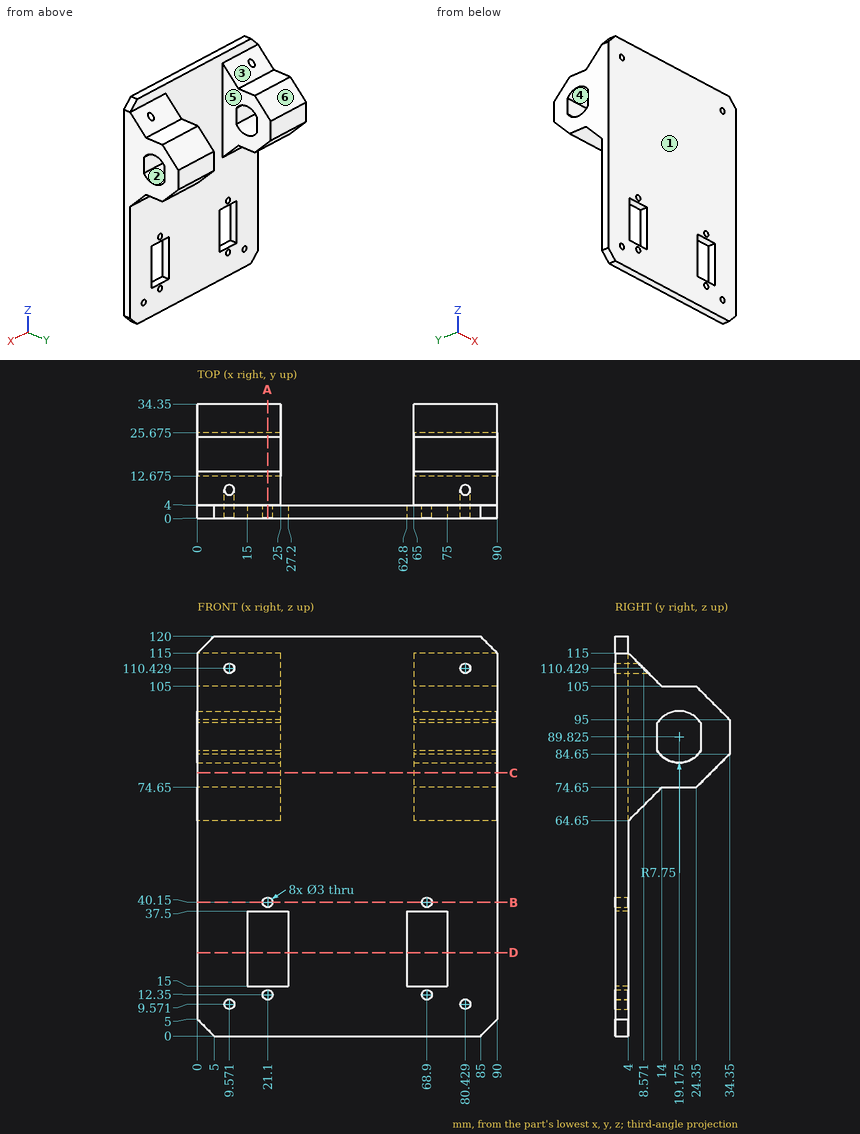
Design review of the part shown in the three views and the two pictorial views. Dimensions are in mm from the part's minimum x, y and z. A direction names the side the tool comes from. Round coordinates to 2 decimals unless told otherwise and drop trailing zeros. Loops run counter-clockwise (first coordinate to the right, second up) from the corner with the lowest first, then second, coordinate; pieces in that order, holes last. Notation, with made-up numbers: (-20.75, 5.5) - (35.25, 5.5) arc R24 ccw to (35.25, 32.5) - close; hole circle Ø9 at (23, -17). An arc over 180 degrees is marked (long way). One line per item, written item: value. Start each with the question number.
Item 1: Take a section at B-B (z = 40.15). Give the boundary of the cut face in (x, y).
Item 2: Take a section at D-D (z = 25). Give the boundary of the cut face in (x, y), plus the area to 3 significant figures.
Item 3: For the marked faces 4, 5 and 6, list the 3-axis set-ups (+Z, -Z, +X, -X, +Y, -Y) from which the entire face can be reached by the end or side of a thin tool; tool diameter is ignored.
Item 4: Clearance check with flat-ended pins moving along their axes: pin 1 Ø2 at (y, z) = (2, 23.5) entering from -X; pin 2 Ø1 at (x, y) = (9.5, 11) entering from +Z; pin 3 Ø3.5 at (x, z) = (80.43, 9.57) entering from +Y; pin 4 Ø11.5 at (x, y) = (16.5, 20) entering from -Z. State where each tip first meets the part, or that it passes through.
Item 5: Take a section at C-C (z = 79). Give the boundary of the cut face in (x, y), plus the area to 4 significant figures.
Item 6: For L1, parallel to Z at x = 21.1, y = 1.9; L2, parallel to Z at x = 23, y = 18.5; L3, parallel to Y at x = 51, z = 69, list the stretches that pass through material, from the lowest coordinate up.
Item 7: The part is to be moulded in two halves that separate along Z. For the marked faces 1, 2 and 3, say which applies: +Z half, -Z half, draft (parallel to the pull), parting line (faces both ways), or undercut.
Item 8: Take a section at A-A (x = 21.1). State how many separate pieces and enclosed holes the cut face has, plus the area to 3 significant figures.
Answer below:
1. outline: (0, 0) - (19.6, 0) - (19.6, 4) - (0, 4) - close; (22.6, 0) - (67.4, 0) - (67.4, 4) - (22.6, 4) - close; (70.4, 0) - (90, 0) - (90, 4) - (70.4, 4) - close
2. outline: (0, 0) - (15, 0) - (15, 4) - (0, 4) - close; (27.2, 0) - (62.8, 0) - (62.8, 4) - (27.2, 4) - close; (75, 0) - (90, 0) - (90, 4) - (75, 4) - close
2. area: 262 mm2
3. face 4: +X, -X
3. face 5: +Z, -Z, +Y
3. face 6: +Z, +X, -X, +Y
4. pin 1: stops at x = 0
4. pin 2: stops at z = 108.5
4. pin 3: stops at y = 4
4. pin 4: stops at z = 74.65
5. outline: (0, 0) - (90, 0) - (90, 28.7) - (65, 28.7) - (65, 4) - (25, 4) - (25, 28.7) - (0, 28.7) - close
5. area: 1,595 mm2
6. L1: z = 0 to 10.85, 13.85 to 15, 37.5 to 38.65, 41.65 to 120
6. L2: z = 74.65 to 82.1, 97.55 to 105
6. L3: y = 0 to 4
7. face 1: draft
7. face 2: undercut
7. face 3: +Z half
8. separate pieces: 4
8. enclosed holes: 1
8. area: 1,110 mm2
